Part model, mm, in its own coordinate system. Face numbers are marked on the shaded views. Give positions to 0.01 mm unless a question says otherwise; leave off trailing zeros. Write each loop counter-clockwise with the first axis right and the second up, starting at its lowest first coordinate (ties: lowest second). Pieces come first, ordered by that corner, then holes. Notation, with made-up numbers: M 66,-5.5 L 112,-5.5 A29 ccw 112,23.5 Z; hole C 60,18.25 d4. An arc over 180 degrees is marked long. Use a Markdown table: item, result. Add a question column.
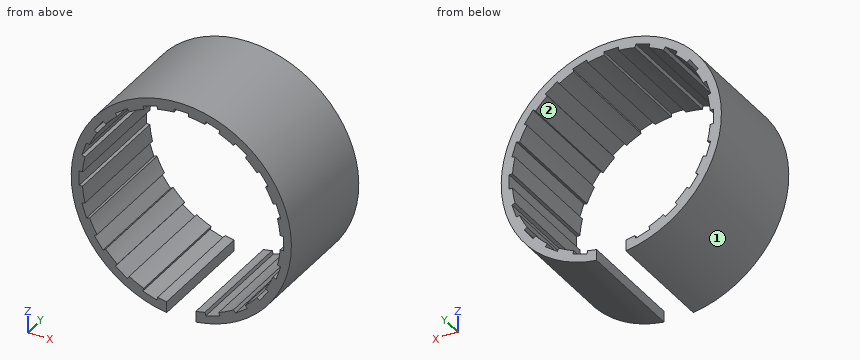
from build123d import *

# Parameters (mm, degrees)
F0_R     = 15
F0_R_2   = 13.5
F1_DEPTH = 15.5
F2_W     = 4
F2_H     = 19.090906
F3_DEPTH = 25
F4_W     = 2
F4_H     = 0.5
F4_W_2   = 0.5
F4_H_2   = 2
F5_DEPTH = 25


with BuildPart() as f1:
    # F0 (on Front) → F1 (new body)
    with BuildSketch(Plane.XZ):
        Circle(F0_R)
        Circle(F0_R_2, mode=Mode.SUBTRACT)
    extrude(amount=F1_DEPTH)

    # F2 (on Top) → F3 (cut)
    with BuildSketch(Plane.XY):
        with Locations((0, -8.067074)):
            Rectangle(F2_W, F2_H)
    extrude(amount=-F3_DEPTH, mode=Mode.SUBTRACT)

    # F4 (on Front) → F5 (cut, symmetric)
    with BuildSketch(Plane.XZ):
        with Locations((0, 13.665518)):
            Rectangle(F4_W, F4_H)
        Polygon((-5.251188, 12.925427), (-5.09668, 12.449899), (-3.194566, 13.067933), (-3.349075, 13.543461), align=None)
        Polygon((-8.988353, 10.670105), (-8.694461, 10.265597), (-7.076427, 11.441167), (-7.370319, 11.845676), align=None)
        Polygon((-11.845676, 7.370319), (-11.441167, 7.076427), (-10.265597, 8.694461), (-10.670105, 8.988353), align=None)
        Polygon((-13.543461, 3.349075), (-13.067933, 3.194566), (-12.449899, 5.09668), (-12.925427, 5.251188), align=None)
        with Locations((-13.665518, 0)):
            Rectangle(F4_W_2, F4_H_2)
        Polygon((-12.925427, -5.251188), (-12.449899, -5.09668), (-13.067933, -3.194566), (-13.543461, -3.349075), align=None)
        Polygon((-10.670105, -8.988353), (-10.265597, -8.694461), (-11.441167, -7.076427), (-11.845676, -7.370319), align=None)
        Polygon((-7.370319, -11.845676), (-7.076427, -11.441167), (-8.694461, -10.265597), (-8.988353, -10.670105), align=None)
        Polygon((-3.349075, -13.543461), (-3.194566, -13.067933), (-5.09668, -12.449899), (-5.251188, -12.925427), align=None)
        with Locations((0, -13.665518)):
            Rectangle(F4_W, F4_H)
        Polygon((5.251188, -12.925427), (5.09668, -12.449899), (3.194566, -13.067933), (3.349075, -13.543461), align=None)
        Polygon((8.988353, -10.670105), (8.694461, -10.265597), (7.076427, -11.441167), (7.370319, -11.845676), align=None)
        Polygon((11.845676, -7.370319), (11.441167, -7.076427), (10.265597, -8.694461), (10.670105, -8.988353), align=None)
        Polygon((13.543461, -3.349075), (13.067933, -3.194566), (12.449899, -5.09668), (12.925427, -5.251188), align=None)
        with Locations((13.665518, 0)):
            Rectangle(F4_W_2, F4_H_2)
        Polygon((12.925427, 5.251188), (12.449899, 5.09668), (13.067933, 3.194566), (13.543461, 3.349075), align=None)
        Polygon((10.670105, 8.988353), (10.265597, 8.694461), (11.441167, 7.076427), (11.845676, 7.370319), align=None)
        Polygon((7.370319, 11.845676), (7.076427, 11.441167), (8.694461, 10.265597), (8.988353, 10.670105), align=None)
        Polygon((3.349075, 13.543461), (3.194566, 13.067933), (5.09668, 12.449899), (5.251188, 12.925427), align=None)
    extrude(amount=F5_DEPTH, both=True, mode=Mode.SUBTRACT)


solid = f1.part
1. Cut at A-A (z = 0). Write the cut outline in (x, y).
2. Flat gauge pins, fed straight in: pin 1 (8 mm diameter, centred on x = -4, y = -8.5, fed in from -Z); pin 2 (2 mm diameter, centred on x = -0.5, y = -5, fed in from -Z); pin 3 (0.5 mm diameter, centred on y = -5, z = 13.5, fed in from +X); pin 4 (10 mm diameter, centred on x = 0.5, z = 5.5, fed in from +Y). Where does each tip first touch, or does it go through?
3. Mould opens along Z. For the marked faces 1 and 2 say: released by +Z, released by -Z, zero draft, split by the parting line, or undercut.
4. Drill centre lines: probe 1 along Z at (x, y) = (8, -9.75); probe 2 along X at (y, z) = (-12.5, 3); probe 3 along X at (y, z) = (-13.25, -4). Where is each one in solid material? Low to high. Write a range as [from, to].
5. Cut at C-C (x = 0). Write the cut outline in (y, z), then the cut area to 3 significant figures.
6. Cut at B-B (x = -4). Write the cut outline in (y, z).
A:
| question | item | result |
|---|---|---|
| 1 | outline | M -15,-15.5 L -13.92,-15.5 L -13.92,0 L -15,0 Z; M 13.92,-15.5 L 15,-15.5 L 15,0 L 13.92,0 Z |
| 2 | pin 1 | stops at z = -14.87 |
| 2 | pin 2 | stops at z = 13.42 |
| 2 | pin 3 | stops at x = 7.03 |
| 2 | pin 4 | passes through |
| 3 | face 1 | split by the parting line |
| 3 | face 2 | undercut |
| 4 | probe 1 | z = [-12.69, -11.39], [11.39, 12.69] |
| 4 | probe 2 | x = [-14.7, -13.16], [13.16, 14.7] |
| 4 | probe 3 | x = [-14.46, -13.33], [13.33, 14.46] |
| 5 | outline | M -15.5,13.92 L 0,13.92 L 0,15 L -15.5,15 Z |
| 5 | area | 16.8 mm² |
| 6 | outline | M -15.5,-14.46 L 0,-14.46 L 0,-13.33 L -15.5,-13.33 Z; M -15.5,13.33 L 0,13.33 L 0,14.46 L -15.5,14.46 Z |
